from build123d import *

# Parameters (mm, degrees)
F0_W     = 42.949088
F0_H     = 77.354542
F1_DEPTH = 12.7
F3_DEPTH = 25.4
F4_W     = 42.949088
F4_H     = 13.854544
F5_DEPTH = 76.2


with BuildPart() as f1:
    # F0 (on Top) → F1 (new body)
    with BuildSketch(Plane.XY):
        Rectangle(F0_W, F0_H)
    extrude(amount=F1_DEPTH)

    # F2 (on face) → F3 (cut)
    with BuildSketch(Plane.XY.offset(12.7)):
        with BuildLine():
            ThreePointArc((21.474544, 0), (0, -21.474544), (-21.474544, 0))
            Line((-21.474544, 0), (-21.474544, -38.677271))
            Line((-21.474544, -38.677271), (21.474544, -38.677271))
            Line((21.474544, -38.677271), (21.474544, 0))
        make_face()
    extrude(amount=-F3_DEPTH, mode=Mode.SUBTRACT)

    # F4 (on face) → F5 (join)
    with BuildSketch(Plane.XY.offset(12.7)):
        with Locations((0, 31.749999)):
            Rectangle(F4_W, F4_H)
    extrude(amount=F5_DEPTH)


solid = f1.part
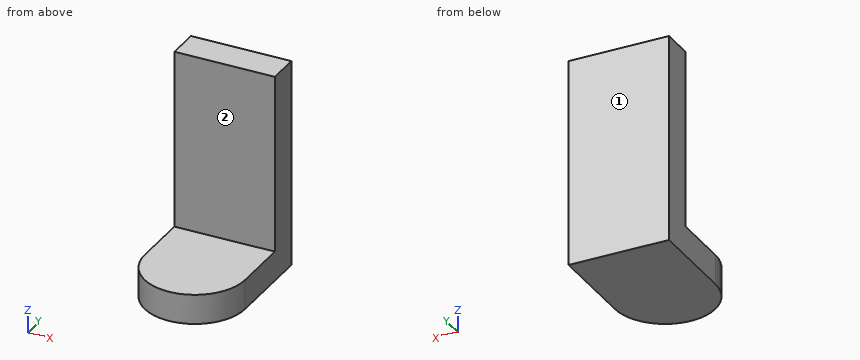
Can you work these out from the model? Positions are in its coordinate system, mm. Face numbers are marked on the shaded views. A direction names the side the tool comes from. Coordinates: 2 decimals unless noted, no trailing zeros. Order: outer loops, then holes, each group sorted by start corner. A loop starts at its lowest first (then second) coordinate and runs counter-clockwise, first axis right, second up. Notation, with made-up numbers: (79, 6) - (93, 6) arc R21 ccw to (93, 37) - close; hole circle Ø1 at (-22.5, 80.5). An arc over 180 degrees is marked (long way). Answer as a JSON object with one key per item and string values. Group by question number.
Q1. I need wall thicknesses on line 1 (Y direction, x = 13, z = 45); line 2 (Z direction, x = 8.5, y = -16); line 3 (Y direction, x = -18, z = 6.5). Which ranges of each line are inside material? Lowest first, please. Write a range as from..to.
Q2. Will these pins go through, and if not, where does the flat tip stop? P1, Ø10, axis at y = 17.5, z = 64, coming from the -X side; P2, Ø1.5, axis at x = 17, z = 22, coming from the -Y side; P3, Ø4, axis at x = -0.5, y = -0.5, coming from the +Z side.
Q3. Imagine slicing it at D-D (x = 7). Please give me the cut outline in (y, z), and give its area (3 significant figures).
Q4. Imagine slicing it at A-A (x = 0). Please give me the cut outline in (y, z), and give its area (3 significant figures).
Q5. Imagine slicing it at C-C (y = 15.5). Please give me the cut outline in (x, z), and give its area (3 significant figures).
Q6. On a 3-axis mill with a long thin cutter (end or side, diameter ignored), from which of +Z, -Z, +X, -X, +Y, -Y can I reach the whole of each face in a straight line? I mean the marked faces 1 and 2. Say none if no direction works.
Q7. Imagine slicing it at B-B (z = 21.5). Please give me the cut outline in (x, y).
Determined:
{
 "1": {"line 1": "y = 24.82..38.68", "line 2": "z = 0..12.7", "line 3": "y = -11.71..38.68"},
 "2": {"P1": "passes through", "P2": "stops at y = 24.82", "P3": "stops at z = 12.7"},
 "3": {"outline": "(-20.3, 0) - (38.68, 0) - (38.68, 88.9) - (24.82, 88.9) - (24.82, 12.7) - (-20.3, 12.7) - close", "area": "1,800 mm2"},
 "4": {"outline": "(-21.47, 0) - (38.68, 0) - (38.68, 88.9) - (24.82, 88.9) - (24.82, 12.7) - (-21.47, 12.7) - close", "area": "1,820 mm2"},
 "5": {"outline": "(-21.47, 0) - (21.47, 0) - (21.47, 12.7) - (-21.47, 12.7) - close", "area": "545 mm2"},
 "6": {"face 1": "+Z, -Z, +X, -X, +Y", "face 2": "+Z, +X, -X, -Y"},
 "7": {"outline": "(-21.47, 24.82) - (21.47, 24.82) - (21.47, 38.68) - (-21.47, 38.68) - close"}
}
